Read the model definition and answer for the solid it produces. Units are mm, in the model's axes. Face numbers are marked on the shaded views. Round coordinates to 2 decimals unless told otherwise and drop trailing zeros. Loops run counter-clockwise (first coordinate to the right, second up) from the corner with the lowest first, then second, coordinate; pieces in that order, holes last. Notation, with made-up numbers: (20.25, 50) -> (32.25, 50) arc R24 ccw to (32.25, 67) -> close; hole circle Ø6 at (0, 34.25). An arc over 180 degrees is marked (long way). Put each result on its own line as item: value.
from build123d import *

# Parameters (mm, degrees)
SKETCH1_R           = 7.366
SKETCH1_R_2         = 1.5875
BOSS_EXTRUDE1_DEPTH = 4.7625
CHAMFER1_SIZE       = 2.3


with BuildPart() as part:
    # Sketch1 → Boss-Extrude1 (new body)
    with BuildSketch(Plane(origin=(0, 0, 0), x_dir=(0, 0, -1), z_dir=(1, 0, 0))):
        with BuildLine():
            Line((4.281323883, 27.486066169), (11.500019866, 12.67082398))
            ThreePointArc((11.500019866, 12.67082398), (11.987341379, 11.987341379), (12.67082398, 11.500019866))
            Line((12.67082398, 11.500019866), (27.486066169, 4.281323883))
            ThreePointArc((27.486066169, 4.281323883), (30.1625, 0), (27.486066169, -4.281323883))
            Line((27.486066169, -4.281323883), (12.67082398, -11.500019866))
            ThreePointArc((12.67082398, -11.500019866), (11.987341379, -11.987341379), (11.500019866, -12.67082398))
            Line((11.500019866, -12.67082398), (4.281323883, -27.486066169))
            ThreePointArc((4.281323883, -27.486066169), (-0.706534615, -30.109799899), (-4.704972325, -26.137998423))
            Line((-4.704972325, -26.137998423), (-7.203117872, -10.211533956))
            ThreePointArc((-7.203117872, -10.211533956), (-8.217337882, -8.217337882), (-10.211533956, -7.203117872))
            Line((-10.211533956, -7.203117872), (-26.137998423, -4.704972325))
            ThreePointArc((-26.137998423, -4.704972325), (-30.109799899, -0.706534615), (-27.486066169, 4.281323883))
            Line((-27.486066169, 4.281323883), (-12.67082398, 11.500019866))
            ThreePointArc((-12.67082398, 11.500019866), (-11.987341379, 11.987341379), (-11.500019866, 12.67082398))
            Line((-11.500019866, 12.67082398), (-4.281323883, 27.486066169))
            ThreePointArc((-4.281323883, 27.486066169), (0, 30.1625), (4.281323883, 27.486066169))
        make_face()
        with Locations(Location((0, 0, 0), (0, 0, 180))):
            Circle(SKETCH1_R, mode=Mode.SUBTRACT)
        with Locations(Location((0, 25.4, 0), (0, 0, 180))):
            Circle(SKETCH1_R_2, mode=Mode.SUBTRACT)
        with Locations(Location((0, 12.5, 0), (0, 0, 180))):
            Circle(SKETCH1_R_2, mode=Mode.SUBTRACT)
        with Locations(Location((12.5, 0, 0), (0, 0, 180))):
            Circle(SKETCH1_R_2, mode=Mode.SUBTRACT)
        with Locations(Location((25.4, 0, 0), (0, 0, 180))):
            Circle(SKETCH1_R_2, mode=Mode.SUBTRACT)
        with Locations(Location((0, -12.5, 0), (0, 0, 180))):
            Circle(SKETCH1_R_2, mode=Mode.SUBTRACT)
        with Locations(Location((0, -25.4, 0), (0, 0, 180))):
            Circle(SKETCH1_R_2, mode=Mode.SUBTRACT)
        with Locations(Location((-12.5, 0, 0), (0, 0, 180))):
            Circle(SKETCH1_R_2, mode=Mode.SUBTRACT)
        with Locations(Location((-25.4, 0, 0), (0, 0, 180))):
            Circle(SKETCH1_R_2, mode=Mode.SUBTRACT)
    extrude(amount=BOSS_EXTRUDE1_DEPTH)

    # Chamfer1
    chamfer1_edges = [part.edges().sort_by_distance(p)[0] for p in [
        (4.7625, 0, -14.0875),
        (4.7625, 12.5, -1.5875),
        (4.7625, 0, 10.9125),
        (4.7625, -12.5, -1.5875),
    ]]
    chamfer(chamfer1_edges, length=CHAMFER1_SIZE)


solid = part.part
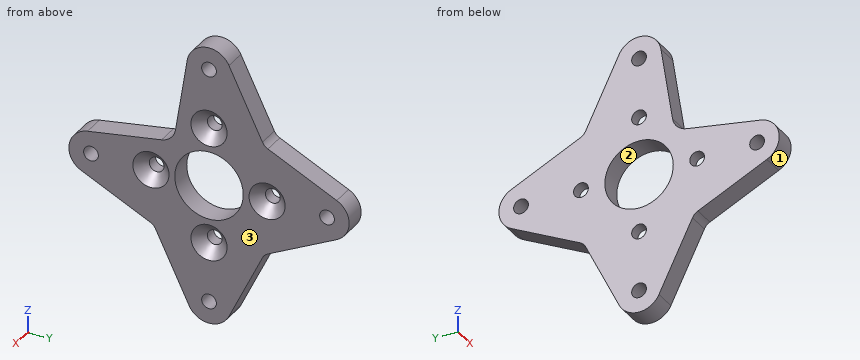
Item 1: Find the intervals of material crossed by line 1 along Y through (x, z) = (0.8, 0); line 2 along Y through (x, z) = (4.1, 2.5); line 3 along Z through (x, y) = (4.1, -14.5), in increasing order.
Derived:
line 1: y = -30.16 to -26.99, -23.81 to -14.09, -10.91 to -7.37, 7.37 to 10.91, 14.09 to 23.81, 26.99 to 30.16
line 2: y = -29.45 to -14.54, -10.46 to -6.93, 6.93 to 10.46, 14.54 to 29.45
line 3: z = -10.61 to -2.53, 2.53 to 6.53
Item 2: The part is cut by section A-A (z = 0). Determine the outline of the cut face in (x, y).
Derived:
outline: (0, -30.16) -> (4.76, -30.16) -> (4.76, -26.99) -> (0, -26.99) -> close; (0, -23.81) -> (4.76, -23.81) -> (4.76, -16.39) -> (2.46, -14.09) -> (0, -14.09) -> close; (0, -10.91) -> (2.46, -10.91) -> (4.76, -8.61) -> (4.76, -7.37) -> (0, -7.37) -> close; (0, 7.37) -> (4.76, 7.37) -> (4.76, 8.61) -> (2.46, 10.91) -> (0, 10.91) -> close; (0, 14.09) -> (2.46, 14.09) -> (4.76, 16.39) -> (4.76, 23.81) -> (0, 23.81) -> close; (0, 26.99) -> (4.76, 26.99) -> (4.76, 30.16) -> (0, 30.16) -> close
Item 3: For a pull along Z with two mould halves and no side action, classify the marked faces 1, 2 and 3 as pulls with the +Z half, pulls with the -Z half, needs draft (parallel to the pull), parting line crosses it, or undercut.
Derived:
face 1: parting line crosses it
face 2: undercut
face 3: needs draft
Item 4: The part is cut by section D-D (y = -24.5). Determine the outline of the cut face in (x, z).
Derived:
outline: (0, -5.74) -> (4.76, -5.74) -> (4.76, -1.31) -> (0, -1.31) -> close; (0, 1.31) -> (4.76, 1.31) -> (4.76, 4.96) -> (0, 4.96) -> close
Item 5: The part is cut by section C-C (z = 25.4). Determine the outline of the cut face in (x, y).
Derived:
outline: (0, -4.82) -> (4.76, -4.82) -> (4.76, -1.59) -> (0, -1.59) -> close; (0, 1.59) -> (4.76, 1.59) -> (4.76, 5.3) -> (0, 5.3) -> close
Item 6: Flat-ended cylindrical pins translate along their axes: pin 1 Ø3 at (y, z) = (0, -12.5) entering from +X; pin 2 Ø4 at (y, z) = (0, 25.4) entering from -X; pin 3 Ø1 at (x, z) = (3, -20.5) entering from -Y; pin 4 Ø3.5 at (y, z) = (0, 12.5) entering from +X (3 decimals). Find the tip coordinate at first contact, or state that the pin passes through.
Derived:
pin 1: passes through
pin 2: stops at x = 0
pin 3: stops at y = -7.93
pin 4: stops at x = 2.625
